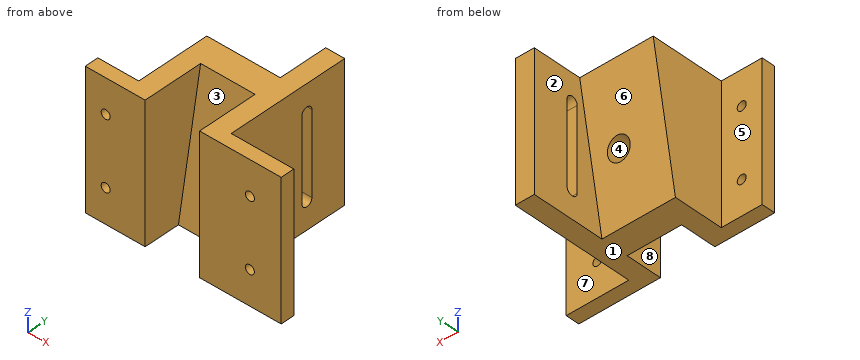
```python
from build123d import *

# Parameters (mm, degrees)
RESSALTO_EXTRUS_O1_DEPTH = 50
CORTE_EXTRUS_O1_DEPTH    = 50
ESBO_O5_R                = 1.65
CORTE_EXTRUS_O2_DEPTH    = 10
ESBO_O7_W                = 27
ESBO_O7_H                = 9.386843201
ESBO_O7_W_2              = 20
ESBO_O7_H_2              = 15
CORTE_EXTRUS_O3_DEPTH    = 84.527706575
ESBO_O8_R                = 4.15
CORTE_EXTRUS_O4_DEPTH    = 77.677309979


with BuildPart() as part:
    # Esboço2 → Ressalto-extrusão1 (new body)
    with BuildSketch(Plane.XY):
        Polygon((0, 0), (30, 0), (30, 5), (7, 5), (7, 50), (0, 50), (0, 32), (-20, 32), (-27, 32), (-27, 5), (-42, 5), (-42, 0), (-20, 0), (-20, 7), (0, 7), align=None)
    extrude(amount=RESSALTO_EXTRUS_O1_DEPTH)

    # Esboço3 → Corte-extrusão1 (cut)
    with BuildSketch(Plane(origin=(7, 0, 0), x_dir=(0, 0, -1), z_dir=(1, 0, 0))):
        with BuildLine():
            Line((-40, 33), (-10, 33))
            ThreePointArc((-10, 33), (-8, 35), (-10, 37))
            Line((-10, 37), (-40, 37))
            ThreePointArc((-40, 37), (-42, 35), (-40, 33))
        make_face()
    extrude(amount=-CORTE_EXTRUS_O1_DEPTH, mode=Mode.SUBTRACT)

    # Esboço5 → Corte-extrusão2 (cut)
    with BuildSketch(Plane(origin=(0, 5, 0), x_dir=(1, 0, 0), z_dir=(0, 1, 0))):
        with Locations(Location((18.5, -37.5, 0), (0, 0, 180))):
            Circle(ESBO_O5_R)
        with Locations(Location((18.5, -12.5, 0), (0, 0, 180))):
            Circle(ESBO_O5_R)
        with Locations(Location((-34.5, -12.5, 0), (0, 0, 180))):
            Circle(ESBO_O5_R)
        with Locations(Location((-34.5, -37.5, 0), (0, 0, 180))):
            Circle(ESBO_O5_R)
    extrude(amount=-CORTE_EXTRUS_O2_DEPTH, mode=Mode.SUBTRACT)

    # Esboço7 → Corte-extrusão3 (cut, through all, along a direction that is not the sketch's normal)
    with BuildSketch(Plane.XY.offset(50)):
        with Locations((-13.5, 36.693421601)):
            Rectangle(ESBO_O7_W, ESBO_O7_H)
        with Locations((-10, 14.5)):
            Rectangle(ESBO_O7_W_2, ESBO_O7_H_2)
    extrude(amount=-CORTE_EXTRUS_O3_DEPTH, dir=(0, 0.1736481776669347, 0.9848077530122074), mode=Mode.SUBTRACT)

    # Esboço8 → Corte-extrusão4 (cut, through all)
    with BuildSketch(Plane(origin=(0, 12.786115246, -2.254537096), x_dir=(1, 0, 0), z_dir=(0, -0.9848077530122075, 0.1736481776669347))):
        with Locations(Location((-10, 27.674982262, 0), (0, 0, 270))):
            Circle(ESBO_O8_R)
    extrude(amount=-CORTE_EXTRUS_O4_DEPTH, mode=Mode.SUBTRACT)


solid = part.part
```
Could you check a few things on this model? Use its own coordinates, in mm. Face numbers are marked on the shaded views. A direction names the side the tool comes from. Round coordinates to 2 decimals unless told otherwise and drop trailing zeros. Loops run counter-clockwise (first coordinate to the right, second up) from the corner with the lowest first, then second, coordinate; pieces in that order, holes last. Notation, with made-up numbers: (47, 38) -> (95, 38) arc R20 ccw to (95, 43) -> close; hole circle Ø6 at (20, 16). An arc over 180 degrees is marked (long way). Put each result on its own line as item: value.
Q1. I want a section at A-A on x = -34.5. Write out the boundary of the cut face in (y, z), and give its area (3 significant figures).
Checks:
outline: (0, 0) -> (5, 0) -> (5, 10.85) -> (0, 10.85) -> close; (0, 14.15) -> (5, 14.15) -> (5, 35.85) -> (0, 35.85) -> close; (0, 39.15) -> (5, 39.15) -> (5, 50) -> (0, 50) -> close
area: 217 mm2
Q2. I want a section at D-D on z = 15. Write out the boundary of the cut face in (x, y).
Checks:
outline: (-42, 0) -> (-20, 0) -> (-20, 15.83) -> (0, 15.83) -> (0, 0) -> (30, 0) -> (30, 5) -> (7, 5) -> (7, 33) -> (0, 33) -> (0, 25.83) -> (-27, 25.83) -> (-27, 5) -> (-42, 5) -> close; (0, 37) -> (7, 37) -> (7, 50) -> (0, 50) -> close
Q3. I want a section at C-C on z = 37.5. Write out the boundary of the cut face in (x, y).
Checks:
outline: (-42, 0) -> (-36.15, 0) -> (-36.15, 5) -> (-42, 5) -> close; (-32.85, 0) -> (-20, 0) -> (-20, 19.8) -> (0, 19.8) -> (0, 0) -> (16.85, 0) -> (16.85, 5) -> (7, 5) -> (7, 33) -> (0, 33) -> (0, 29.8) -> (-27, 29.8) -> (-27, 5) -> (-32.85, 5) -> close; (0, 37) -> (7, 37) -> (7, 50) -> (0, 50) -> close; (20.15, 0) -> (30, 0) -> (30, 5) -> (20.15, 5) -> close
Q4. Please list where these lines run through material, in increasing order: line 1 (Z direction, x = -34.5, y = 3.8); line 2 (X direction, y = 6.5, z = 16); line 3 (Y direction, x = 2, z = 23.5). Write a range as from..to.
Checks:
line 1: 0..10.85, 14.15..35.85, 39.15..50
line 2: -27..-20, 0..7
line 3: 0..33, 37..50
Q5. For pin 1 Ø12 at (x, z) = (-34.5, 24.5) entering from +Y; pin 2 Ø6 at (y, z) = (44.5, 13) entering from +X; pin 3 Ø13.5 at (y, z) = (13, 20) entering from -X, each with a flat end and sliding along its axis, tell me the tip position at first contact or that it passes through.
Checks:
pin 1: y = 5
pin 2: x = 7
pin 3: x = -27
Q6. I want a section at B-B on y = 35. Write out the boundary of the cut face in (x, z).
Checks:
outline: (0, 0) -> (7, 0) -> (7, 8) -> (0, 8) -> close; (0, 42) -> (7, 42) -> (7, 50) -> (0, 50) -> close
Q7. Which directions (+Z, -Z, +X, -X, +Y, -Y) give clear straight access to the entire face, cutting with the end or side of a thin tool? Please do the marked faces 5, 6, 7 and 8.
Checks:
face 5: +Z, -Z, -X, +Y
face 6: -Z, -X, +Y
face 7: +Z, -Z, +X, +Y
face 8: +Z, -Y
Q8. Thinking about a two-plate mould opening in Z: for the marked faces 1, 2, 3 and 4, which applies, pulls with the +Z half, pulls with the -Z half, needs draft (parallel to the pull), parting line crosses it, or undercut?
Checks:
face 1: pulls with the -Z half
face 2: needs draft
face 3: pulls with the +Z half
face 4: undercut
